from build123d import *

# Parameters (mm, degrees)
SKETCH_1_W      = 4.1
SKETCH_1_H      = 15.1
SKETCH_1_H_2    = 25
EXTRUDE_1_DEPTH = 4


with BuildPart() as part:
    # ｽｹｯﾁ1 → ﾎﾞｽ - 押し出し1 (new body)
    with BuildSketch(Plane(origin=(0, 0, 0), x_dir=(0, 1, 0), z_dir=(0, 0, 1))):
        Polygon((165, 60), (165, 63.9), (145, 63.9), (145, 60), (97.5, 60), (97.5, 63.9), (77.5, 63.9), (77.5, 60), (30, 60), (30, 63.9), (10, 63.9), (10, 60), (0, 60), (0, 45), (-3.9, 45), (-3.9, 15), (0, 15), (0, 0), (10, 0), (10, -3.9), (30, -3.9), (30, 0), (77.5, 0), (77.5, -3.9), (97.5, -3.9), (97.5, 0), (145, 0), (145, -3.9), (165, -3.9), (165, 0), (175, 0), (175, 60), align=None)
        with Locations((118, 47.5)):
            Rectangle(SKETCH_1_W, SKETCH_1_H, mode=Mode.SUBTRACT)
        with Locations((118, 12.5)):
            Rectangle(SKETCH_1_W, SKETCH_1_H, mode=Mode.SUBTRACT)
        with Locations((169, 30)):
            Rectangle(SKETCH_1_W, SKETCH_1_H_2, mode=Mode.SUBTRACT)
    extrude(amount=EXTRUDE_1_DEPTH)


solid = part.part
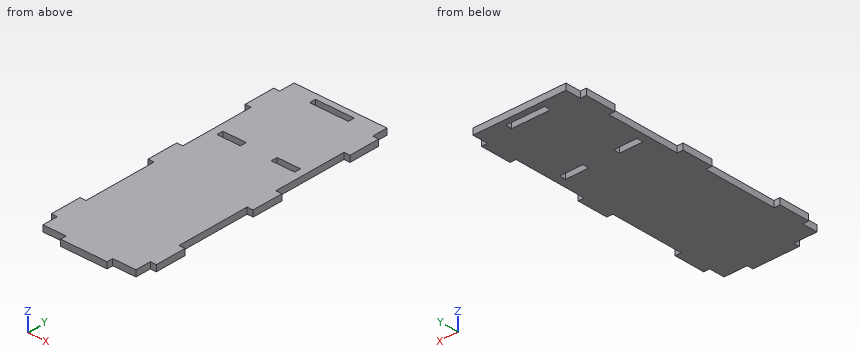
Could you check a few things on this model? Use its own coordinates, in mm. Give positions to 0.01 mm unless a question says otherwise; leave off trailing zeros. Order: outer loops, then holes, each group sorted by start corner. A loop starts at its lowest first (then second) coordinate and runs counter-clockwise, first axis right, second up.
1. Suppose I cut it at C-C (y = 38). List the corners of the cut face in (x, z) for me, plus the area to 3 significant figures.
2. Suppose I cut it at A-A (x = -31.5). List the corners of the cut face in (y, z) for me.
3. I need wall thicknesses on L1, parallel to Y at x = -39.5, z = 3.1; L2, parallel to Y at x = -51, z = 2.9; L3, parallel to X at y = 56.5, z = 2.8. Which ranges of each line are inside material? Lowest first, please.
4. Will these pins go through, and if not, where does the flat tip stop? P1, Ø1.2, axis at x = -51, z = 1, coming from the -Y side; P2, Ø1, axis at y = 71, z = 2.5, coming from the -X side; P3, Ø2, axis at y = 118, z = 1.5, coming from the +X side.
5. Suppose I cut it at B-B (z = 3.3). Give the number of separate pieces and of enclosed holes in the cut face, plus the area to 3 significant figures.
Solved:
1. outline: (-60, 0) - (0, 0) - (0, 4) - (-60, 4) - close
1. area: 240 mm2
2. outline: (-3.9, 0) - (166.95, 0) - (166.95, 4) - (-3.9, 4) - close; (171.05, 0) - (175, 0) - (175, 4) - (171.05, 4) - close
3. L1: y = -3.9 to 166.95, 171.05 to 175
3. L2: y = 0 to 115.95, 120.05 to 175
3. L3: x = -60 to 0
4. P1: stops at y = 0
4. P2: stops at x = -60
4. P3: stops at x = 0
5. separate pieces: 1
5. enclosed holes: 3
5. area: 10,900 mm2
